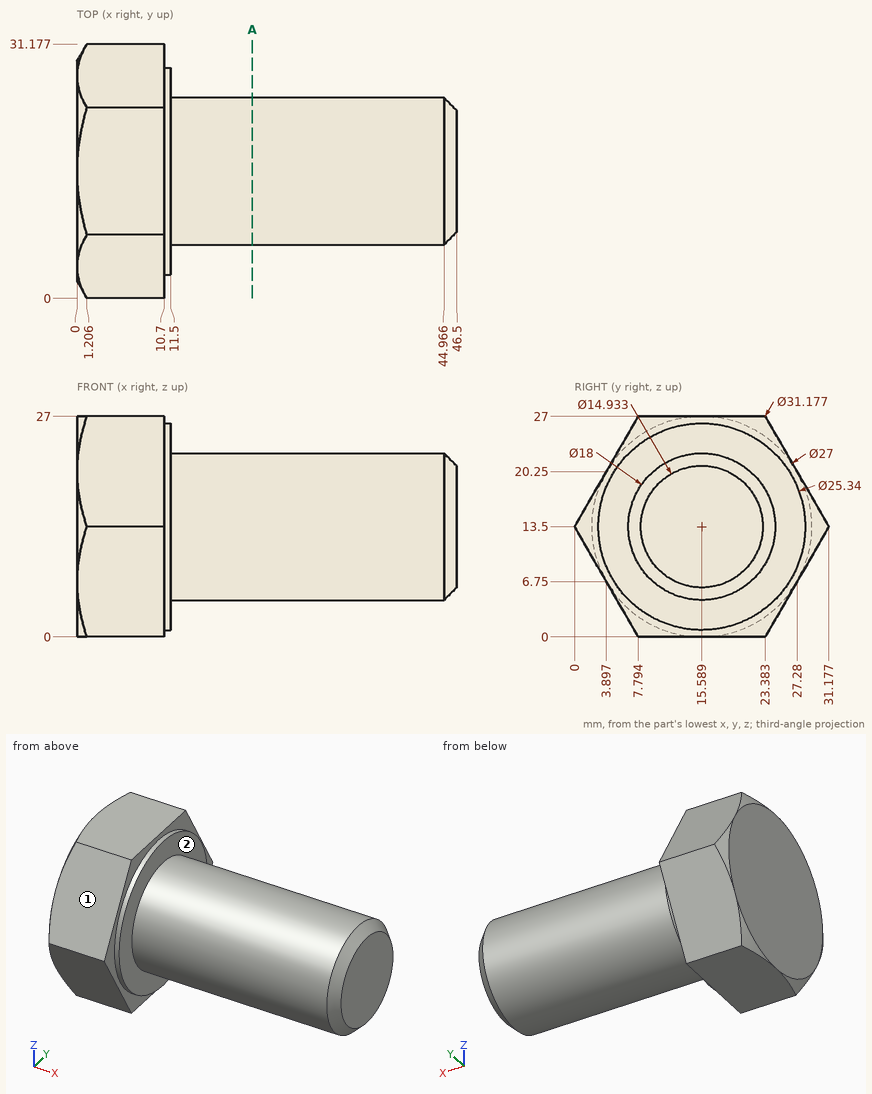
Check sheet for the drawn part. Datum: minimum x, y, z corner. Units: mm. A direction names the side the tool comes from. Give positions to 0.01 mm unless a question says otherwise; leave off trailing zeros. Write each loop counter-clockwise with the first axis right and the second up, starting at its lowest first coordinate (ties: lowest second). Pieces come first, ordered by that corner, then holes. Notation, with made-up numbers: M 16,65.5 L 45,65.5 A22 cw 45,86.5 Z; hole C 67,-2 d5. An arc over 180 degrees is marked long. One line per question, with ' | ' between items.
1) Thickness scan on line 1 along X through (y, z) = (5, 11.5); line 2 along X through (y, z) = (3.5, 18.5); line 3 along Z through (x, y) = (16.5, 15.5). Record the ranges inside material, lowest first. Write a range as [from, to].
Result:
line 1: x = [0, 11.5] | line 2: x = [0, 10.7] | line 3: z = [4.5, 22.5]
2) Section check A-A on x = 21.5. Enter the section's corners in (y, z).
Result:
outline: C 15.59,13.5 d18
3) Gauge pin test, flat ends, axial feed: pin 1 Ø1 at (x, z) = (35, 20) entering from +Y (1 decimal); pin 2 Ø10 at (x, z) = (37, 18) entering from +Y; pin 3 Ø1 at (x, z) = (28, 14) entering from -Y. Record the tip position at first contact, or that the pin passes through.
Result:
pin 1: stops at y = 22.3 | pin 2: stops at y = 24.59 | pin 3: stops at y = 6.59
4) Set-up check for the marked faces 1 and 2: record each of +Z, -Z, +X, -X, +Y, -Y from which the full face is reachable in a straight line by a thin tool's end or side.
Result:
face 1: +Z, +X, -X, -Y | face 2: +X
